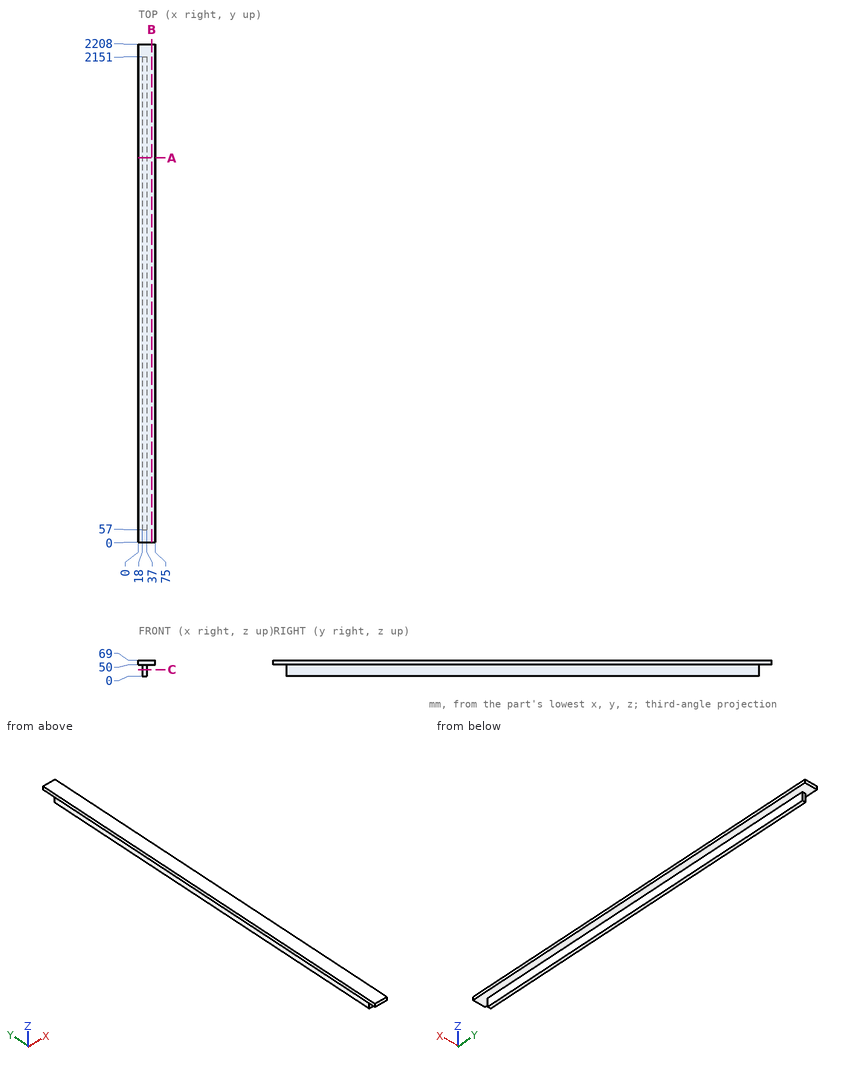
Design review of the part shown in the three views and the two pictorial views. Dimensions are in mm from the part's minimum x, y and z. Give positions to 0.01 mm unless a question says otherwise; leave off trailing zeros. Order: outer loops, then holes, each group sorted by start corner. A loop starts at its lowest first (then second) coordinate and runs counter-clockwise, first axis right, second up. Notation, with made-up numbers: (-12.75, 28) -> (45.25, 28) arc R14 cw to (45.25, 38) -> close; hole circle Ø8 at (71, 47.25). An arc over 180 degrees is marked (long way). Write each question's results on one line, items separated by ' | '. Start each with the question number.
Q1. For pin 1 (5.5 mm diameter, centred on x = 31.5, z = 20, fed in from -Y); pin 2 (3 mm diameter, centred on y = 1151.5, z = 46, fed in from +X); pin 3 (6 mm diameter, centred on y = 973, z = 13, fed in from -X), all flat-tipped, find the tip position at first contact; note any pin that passes through.
Q2. Add section A-A on y = 1703.5. Give the boundary of the cut face in (x, z), and give its area (4 significant figures).
Q3. Add section B-B on x = 59. Give the boundary of the cut face in (y, z).
Q4. Add section C-C on z = 28.5. Give the boundary of the cut face in (x, y), and give its area (3 significant figures).
Q5. Wall thickness on L1, parallel to X at y = 1902, z = 49; L2, parallel to Z at x = 52, y = 148: over which ranges is each line inside the solid? List them lowest first. Write a range as from..to.
Found:
1) pin 1: stops at y = 57 | pin 2: stops at x = 37 | pin 3: stops at x = 18
2) outline: (0, 50) -> (18, 50) -> (18, 0) -> (37, 0) -> (37, 50) -> (75, 50) -> (75, 69) -> (0, 69) -> close | area: 2,375 mm2
3) outline: (0, 50) -> (2208, 50) -> (2208, 69) -> (0, 69) -> close
4) outline: (18, 57) -> (37, 57) -> (37, 2151) -> (18, 2151) -> close | area: 39,800 mm2
5) L1: x = 18..37 | L2: z = 50..69
